```python
from build123d import *

# Parameters (mm, degrees)
BOSS_EXTRUDE1_DEPTH = 123.825
CUT_EXTRUDE1_REACH  = 40.1
SKETCH3_R           = 3.302
CUT_EXTRUDE2_REACH  = 40.1
SKETCH4_R           = 3.302


with BuildPart() as part:
    # Sketch2 → Boss-Extrude1 (new body, symmetric)
    with BuildSketch(Plane.XY):
        with BuildLine():
            Line((-19.05, -19.05), (19.05, -19.05))
            Line((19.05, -19.05), (19.05, 19.05))
            Line((19.05, 19.05), (16.66875, 19.05))
            ThreePointArc((16.66875, 19.05), (14.984951977, 18.352548023), (14.2875, 16.66875))
            Line((14.2875, 16.66875), (14.2875, -9.5123))
            ThreePointArc((14.2875, -9.5123), (12.888876302, -12.888876302), (9.5123, -14.2875))
            Line((9.5123, -14.2875), (-16.66875, -14.2875))
            ThreePointArc((-16.66875, -14.2875), (-18.352548023, -14.984951977), (-19.05, -16.66875))
            Line((-19.05, -16.66875), (-19.05, -19.05))
        make_face()
    extrude(amount=BOSS_EXTRUDE1_DEPTH, both=True)

    # Sketch3 → Cut-Extrude1 (cut, up to next)
    with BuildSketch(Plane(origin=(19.05, 0, 0), x_dir=(0, 0, -1), z_dir=(1, 0, 0)), mode=Mode.PRIVATE) as cut_extrude1_sk1:
        with Locations((111.125, -6.35)):
            Circle(SKETCH3_R)
    cut_extrude1_tool1 = extrude(cut_extrude1_sk1.sketch, amount=-CUT_EXTRUDE1_REACH, mode=Mode.PRIVATE) & part.part
    add(cut_extrude1_tool1.solids().sort_by_distance((19.05, -6.35, -111.125))[0], mode=Mode.SUBTRACT)
    # Sketch3 → Cut-Extrude1 (cut, up to next)
    with BuildSketch(Plane(origin=(19.05, 0, 0), x_dir=(0, 0, -1), z_dir=(1, 0, 0)), mode=Mode.PRIVATE) as cut_extrude1_sk2:
        with Locations((66.675, -6.35)):
            Circle(SKETCH3_R)
    cut_extrude1_tool2 = extrude(cut_extrude1_sk2.sketch, amount=-CUT_EXTRUDE1_REACH, mode=Mode.PRIVATE) & part.part
    add(cut_extrude1_tool2.solids().sort_by_distance((19.05, -6.35, -66.675))[0], mode=Mode.SUBTRACT)
    # Sketch3 → Cut-Extrude1 (cut, up to next)
    with BuildSketch(Plane(origin=(19.05, 0, 0), x_dir=(0, 0, -1), z_dir=(1, 0, 0)), mode=Mode.PRIVATE) as cut_extrude1_sk3:
        with Locations((22.225, -6.35)):
            Circle(SKETCH3_R)
    cut_extrude1_tool3 = extrude(cut_extrude1_sk3.sketch, amount=-CUT_EXTRUDE1_REACH, mode=Mode.PRIVATE) & part.part
    add(cut_extrude1_tool3.solids().sort_by_distance((19.05, -6.35, -22.225))[0], mode=Mode.SUBTRACT)
    # Sketch3 → Cut-Extrude1 (cut, up to next)
    with BuildSketch(Plane(origin=(19.05, 0, 0), x_dir=(0, 0, -1), z_dir=(1, 0, 0)), mode=Mode.PRIVATE) as cut_extrude1_sk4:
        with Locations((-22.225, -6.35)):
            Circle(SKETCH3_R)
    cut_extrude1_tool4 = extrude(cut_extrude1_sk4.sketch, amount=-CUT_EXTRUDE1_REACH, mode=Mode.PRIVATE) & part.part
    add(cut_extrude1_tool4.solids().sort_by_distance((19.05, -6.35, 22.225))[0], mode=Mode.SUBTRACT)
    # Sketch3 → Cut-Extrude1 (cut, up to next)
    with BuildSketch(Plane(origin=(19.05, 0, 0), x_dir=(0, 0, -1), z_dir=(1, 0, 0)), mode=Mode.PRIVATE) as cut_extrude1_sk5:
        with Locations((-66.675, -6.35)):
            Circle(SKETCH3_R)
    cut_extrude1_tool5 = extrude(cut_extrude1_sk5.sketch, amount=-CUT_EXTRUDE1_REACH, mode=Mode.PRIVATE) & part.part
    add(cut_extrude1_tool5.solids().sort_by_distance((19.05, -6.35, 66.675))[0], mode=Mode.SUBTRACT)
    # Sketch3 → Cut-Extrude1 (cut, up to next)
    with BuildSketch(Plane(origin=(19.05, 0, 0), x_dir=(0, 0, -1), z_dir=(1, 0, 0)), mode=Mode.PRIVATE) as cut_extrude1_sk6:
        with Locations((-111.125, -6.35)):
            Circle(SKETCH3_R)
    cut_extrude1_tool6 = extrude(cut_extrude1_sk6.sketch, amount=-CUT_EXTRUDE1_REACH, mode=Mode.PRIVATE) & part.part
    add(cut_extrude1_tool6.solids().sort_by_distance((19.05, -6.35, 111.125))[0], mode=Mode.SUBTRACT)

    # Sketch4 → Cut-Extrude2 (cut, up to next)
    with BuildSketch(Plane.XZ.offset(19.05), mode=Mode.PRIVATE) as cut_extrude2_sk1:
        with Locations((0, -92.075)):
            Circle(SKETCH4_R)
    cut_extrude2_tool1 = extrude(cut_extrude2_sk1.sketch, amount=-CUT_EXTRUDE2_REACH, mode=Mode.PRIVATE) & part.part
    add(cut_extrude2_tool1.solids().sort_by_distance((0, -19.05, -92.075))[0], mode=Mode.SUBTRACT)
    # Sketch4 → Cut-Extrude2 (cut, up to next)
    with BuildSketch(Plane.XZ.offset(19.05), mode=Mode.PRIVATE) as cut_extrude2_sk2:
        with Locations((0, -46.355)):
            Circle(SKETCH4_R)
    cut_extrude2_tool2 = extrude(cut_extrude2_sk2.sketch, amount=-CUT_EXTRUDE2_REACH, mode=Mode.PRIVATE) & part.part
    add(cut_extrude2_tool2.solids().sort_by_distance((0, -19.05, -46.355))[0], mode=Mode.SUBTRACT)
    # Sketch4 → Cut-Extrude2 (cut, up to next)
    with BuildSketch(Plane.XZ.offset(19.05), mode=Mode.PRIVATE) as cut_extrude2_sk3:
        with Locations((0, -0.635)):
            Circle(SKETCH4_R)
    cut_extrude2_tool3 = extrude(cut_extrude2_sk3.sketch, amount=-CUT_EXTRUDE2_REACH, mode=Mode.PRIVATE) & part.part
    add(cut_extrude2_tool3.solids().sort_by_distance((0, -19.05, -0.635))[0], mode=Mode.SUBTRACT)
    # Sketch4 → Cut-Extrude2 (cut, up to next)
    with BuildSketch(Plane.XZ.offset(19.05), mode=Mode.PRIVATE) as cut_extrude2_sk4:
        with Locations((0, 45.085)):
            Circle(SKETCH4_R)
    cut_extrude2_tool4 = extrude(cut_extrude2_sk4.sketch, amount=-CUT_EXTRUDE2_REACH, mode=Mode.PRIVATE) & part.part
    add(cut_extrude2_tool4.solids().sort_by_distance((0, -19.05, 45.085))[0], mode=Mode.SUBTRACT)
    # Sketch4 → Cut-Extrude2 (cut, up to next)
    with BuildSketch(Plane.XZ.offset(19.05), mode=Mode.PRIVATE) as cut_extrude2_sk5:
        with Locations((0, 90.805)):
            Circle(SKETCH4_R)
    cut_extrude2_tool5 = extrude(cut_extrude2_sk5.sketch, amount=-CUT_EXTRUDE2_REACH, mode=Mode.PRIVATE) & part.part
    add(cut_extrude2_tool5.solids().sort_by_distance((0, -19.05, 90.805))[0], mode=Mode.SUBTRACT)


solid = part.part
```
Read the model definition and answer for the solid it produces. Units are mm, in the model's axes. A direction names the side the tool comes from. Coordinates: 2 decimals unless noted, no trailing zeros. Answer as a JSON object with one key per item and string values. Group by question number.
1. Consider L1, parallel to Z at x = 0, y = -16.5 (3 decimals); L2, parallel to X at y = -16.5, z = 102.5; L3, parallel to X at y = -0.5, z = -99. Determine where each line is inside the solid, lowest interval first. Write a range as [from, to].
2. Which of the six approach directions +Z, -Z, +X, -X, +Y, -Y give full straight-line access (tool end or side, diameter ignored) to faces 1 (the cylindrical face through (16.701, -9.573, 22.941)), 2 (the flat face through (-3, -14.288, 2))?
3. A cutting plane is placed at A-A (y = -6.35). Give the number of separate pieces and of enclosed holes in the cut face, plus the area to 3 significant figures.
4. Each of these flat-tipped pins is pushed along its axis until it touches: P1, Ø8.5, axis at x = 0, z = 45.085, coming from the +Y side; P2, Ø6, axis at y = -6.35, z = -22.225, coming from the -X side; P3, Ø7.5, axis at y = -6.35, z = 111.125, coming from the +X side; P4, Ø10.5, axis at y = -6.35, z = -66.675, coming from the -X side. Where does it stop, or does it pass through?
5. The mould has two halves that part along X. Classify faces 3 (the cylindrical face through (16.701, -5.358, -25.375)), 4 (the cylindrical face through (12.93, -12.85, 1.73)), 5 (the cylindrical face through (3.15, -16.7, 0.36)): +X half, -X half, draft (parallel to the pull), parting line (faces both ways), or undercut.
Worked out:
{
 "1": {"L1": "z = [-123.825, -95.377], [-88.773, -49.657], [-43.053, -3.937], [2.667, 41.783], [48.387, 87.503], [94.107, 123.825]", "L2": "x = [-19.04, 19.05]", "L3": "x = [14.29, 19.05]"},
 "2": {"face 1": "+X, -X", "face 2": "+Z, -Z, -X, +Y"},
 "3": {"separate pieces": "7", "enclosed holes": "0", "area": "991 mm²"},
 "4": {"P1": "stops at y = -14.29", "P2": "passes through", "P3": "stops at x = 19.05", "P4": "stops at x = 13.81"},
 "5": {"face 3": "draft", "face 4": "-X half", "face 5": "undercut"}
}
